```python
from build123d import *

# Parameters (mm, degrees)
SKETCH2_R           = 16.7005
SKETCH2_R_2         = 13.3223
BOSS_EXTRUDE1_DEPTH = 457.2


with BuildPart() as part:
    # Sketch2 → Boss-Extrude1 (new body)
    with BuildSketch(Plane.XY):
        Circle(SKETCH2_R)
        Circle(SKETCH2_R_2, mode=Mode.SUBTRACT)
    extrude(amount=BOSS_EXTRUDE1_DEPTH)

    # Sketch3 → Cut-Revolve2 (revolve, cut)
    with BuildSketch(Plane(origin=(0, 0, 0), x_dir=(0, 0, -1), z_dir=(1, 0, 0)), mode=Mode.PRIVATE) as cut_revolve2_sk:
        Polygon((0, 21.813584822), (-19.05, 21.813584822), (-19.05, 16.7005), (-19.05, 15.869250272), (0, 15.126208453), align=None)
        Polygon((-457.2, 15.126208453), (-457.2, 21.813584822), (-438.15, 21.813584822), (-438.15, 16.7005), (-438.15, 15.869250272), align=None)
    revolve(cut_revolve2_sk.sketch.rotate(Axis((0, 0, 228.6), (0, 0, -1)), 180), axis=Axis((0, 0, 228.6), (0, 0, -1)), mode=Mode.SUBTRACT)


solid = part.part
```
Geometry: final body of the model. Coordinates: model frame, mm. A direction names the side the tool comes from. Round coordinates to 2 decimals unless told otherwise and drop trailing zeros. Write each loop counter-clockwise with the first axis right and the second up, starting at its lowest first coordinate (ties: lowest second). Pieces come first, ordered by that corner, then holes. Notation, with made-up numbers: M 45,2 L 96,2 A19 ccw 96,10 Z; hole C 5.5,37 d2. An arc over 180 degrees is marked long. Answer in a Markdown table with one row per item. Add a question column.
(1) Cut plane A-A, the plane x = 0. Return the cut outline in (y, z), then the cut area to 3 significant figures.
(2) Contact query for flat-ended pins moving along their axis: pin 1 (12 mm diameter, centred on x = -12.5, z = 373.5, fed in from -Y); pin 2 (4 mm diameter, centred on x = -4, z = 188, fed in from +Y); pin 3 (4 mm diameter, centred on x = 7.5, z = 237.5, fed in from +Y). Output: stop coordinate, or through.
(3) Reachability of faces 1 (the face through (6, 15, 438.15)), 2 (the face through (6, -15, 19.05)), 3 (the face through (12.707, 4.002, 225.4)) from +Z, -Z, +X, -X, +Y, -Y: full face, straight path, thin tool, end or side. Return the list, or none.
(4) Ray query, L1, parallel to Y at x = 0, z = 299; L2, parallel to X at y = -1.5, z = 34.5; L3, parallel to X at y = -3.5, z = 54. Return the intervals inside material, ascending.
(5) Cut plane C-C, the plane z = 390. Return the cut outline in (x, y), then the cut area to 3 significant figures.
Established:
| question | item | result |
|---|---|---|
| 1 | outline | M -16.7,19.05 L -15.87,19.05 L -15.13,0 L -13.32,0 L -13.32,457.2 L -15.13,457.2 L -15.87,438.15 L -16.7,438.15 Z; M 13.32,0 L 15.13,0 L 15.87,19.05 L 16.7,19.05 L 16.7,438.15 L 15.87,438.15 L 15.13,457.2 L 13.32,457.2 Z |
| 1 | area | 3,000 mm² |
| 2 | pin 1 | y = -15.38 |
| 2 | pin 2 | y = 16.58 |
| 2 | pin 3 | y = 15.77 |
| 3 | face 1 | +Z |
| 3 | face 2 | -Z |
| 3 | face 3 | +Z, -Z |
| 4 | L1 | -16.7 to -13.32, 13.32 to 16.7 |
| 4 | L2 | -16.63 to -13.24, 13.24 to 16.63 |
| 4 | L3 | -16.33 to -12.85, 12.85 to 16.33 |
| 5 | outline | C 0,0 d33.4; hole C 0,0 d26.64 |
| 5 | area | 319 mm² |
